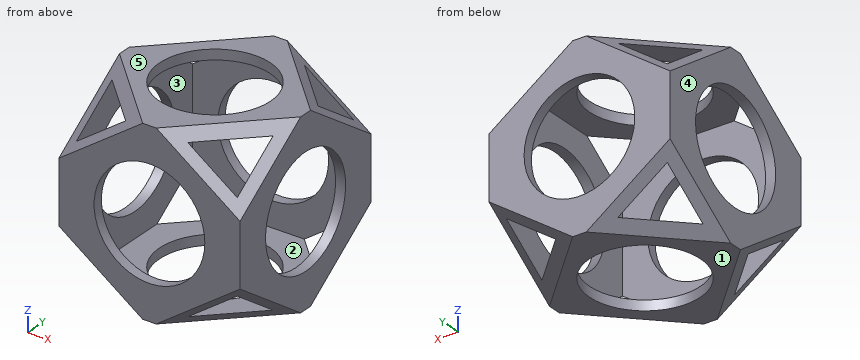
from build123d import *

# Parameters (mm, degrees)
PAD001_DEPTH            = 35
PAD_DEPTH               = 35
CYLINDER002_R           = 27.5
CYLINDER002_DEPTH       = 90
CYLINDER002_PITCH_ANGLE = 90
CYLINDER001_R           = 27.5
CYLINDER001_DEPTH       = 90
CYLINDER001_ROLL_ANGLE  = 90
CYLINDER_R              = 27.5
CYLINDER_DEPTH          = 90
BOX001_W                = 80
BOX001_H                = 80
BOX001_DEPTH            = 80
BOX_W                   = 90
BOX_H                   = 90
BOX_DEPTH               = 90


with BuildPart() as pad001:
    # Sketch001 → Pad001 (new body, symmetric)
    with BuildSketch(Plane(origin=(0, 0, 0), x_dir=(0.707107, -0.707107, 0), z_dir=(-0.707107, -0.707107, 0))):
        Polygon((-65, 14.195959), (-65, 50), (-29.195959, 50), align=None)
        Polygon((29.195959, 50), (65, 50), (65, 14.195959), align=None)
        Polygon((-65, -14.195959), (-65, -50), (-29.195959, -50), align=None)
        Polygon((29.195959, -50), (65, -50), (65, -14.195959), align=None)
    extrude(amount=PAD001_DEPTH, both=True)


with BuildPart() as pad:
    # Sketch → Pad (new body, symmetric)
    with BuildSketch(Plane(origin=(0, 0, 0), x_dir=(0.707107, 0.707107, 0), z_dir=(0.707107, -0.707107, 0))):
        Polygon((-65, 14.195959), (-65, 50), (-29.195959, 50), align=None)
        Polygon((29.195959, 50), (65, 50), (65, 14.195959), align=None)
        Polygon((-65, -14.195959), (-65, -50), (-29.195959, -50), align=None)
        Polygon((29.195959, -50), (65, -50), (65, -14.195959), align=None)
    extrude(amount=PAD_DEPTH, both=True)


with BuildPart() as cylinder002:
    # Cylinder002 → Cylinder002 (new body)
    with BuildSketch(Plane.XY):
        Circle(CYLINDER002_R)
    extrude(amount=CYLINDER002_DEPTH)


with BuildPart() as cylinder002_1:
    # Cylinder002 pitch: moved
    add(cylinder002.part.rotate(Axis((0, 0, 0), (0, 1, 0)), CYLINDER002_PITCH_ANGLE))


with BuildPart() as cylinder002_2:
    # Cylinder002 placement: moved
    add(cylinder002_1.part.moved(Location((-45, 0, 0))))


with BuildPart() as cylinder001:
    # Cylinder001 → Cylinder001 (new body)
    with BuildSketch(Plane.XY):
        Circle(CYLINDER001_R)
    extrude(amount=CYLINDER001_DEPTH)


with BuildPart() as cylinder001_1:
    # Cylinder001 roll: moved
    add(cylinder001.part.rotate(Axis((0, 0, 0), (1, 0, 0)), CYLINDER001_ROLL_ANGLE))


with BuildPart() as cylinder001_2:
    # Cylinder001 placement: moved
    add(cylinder001_1.part.moved(Location((0, 45, 0))))


with BuildPart() as cylinder:
    # Cylinder → Cylinder (new body)
    with BuildSketch(Plane.XY.offset(-45)):
        Circle(CYLINDER_R)
    extrude(amount=CYLINDER_DEPTH)


with BuildPart() as obj1:
    # Box001 → Box001 (new body)
    with BuildSketch(Plane(origin=(-40, -40, -40), x_dir=(1, 0, 0), z_dir=(0, 0, 1))):
        with Locations((40, 40)):
            Rectangle(BOX001_W, BOX001_H)
    extrude(amount=BOX001_DEPTH)


with BuildPart() as cut005:
    # Box → Box (new body)
    with BuildSketch(Plane(origin=(-45, -45, -45), x_dir=(1, 0, 0), z_dir=(0, 0, 1))):
        with Locations((45, 45)):
            Rectangle(BOX_W, BOX_H)
    extrude(amount=BOX_DEPTH)

    # Cut: cut obj1
    add(obj1.part, mode=Mode.SUBTRACT)

    # Cut001: cut Cylinder
    add(cylinder.part, mode=Mode.SUBTRACT)

    # Cut002: cut Cylinder001
    add(cylinder001_2.part, mode=Mode.SUBTRACT)

    # Cut003: cut Cylinder002
    add(cylinder002_2.part, mode=Mode.SUBTRACT)

    # Cut004: cut Pad
    add(pad.part, mode=Mode.SUBTRACT)

    # Cut005: cut Pad001
    add(pad001.part, mode=Mode.SUBTRACT)


solid = cut005.part
Geometry: final body of the model. Coordinates: model frame, mm. Face numbers are marked on the shaded views. A direction names the side the tool comes from. Coordinates: 2 decimals unless noted, no trailing zeros. Order: outer loops, then holes, each group sorted by start corner. A loop starts at its lowest first (then second) coordinate and runs counter-clockwise, first axis right, second up. Notation, with made-up numbers: M 6.25,-25 L 30.25,-25 A20 ccw 30.25,-21 Z; hole C -13.75,13.25 d3. An arc over 180 degrees is marked long. One line per question, with ' | ' between items. Start each with the question number.
Item 1: Set-up query: the marked faces 1 and 2. Return all of +Z, -Z, +X, -X, +Y, -Y with unobstructed straight access to the full face (end or side cutting, diameter ignored); none if empty.
Item 2: Draft query along X for the marked faces 3, 4 and 5. Return one class per face: released by +X, released by -X, zero draft, split by the parting line, or undercut.
Item 3: Cut plane C-C, the plane y = 38. Return the cut outline in (x, z).
Item 4: Cut plane A-A, the plane x = 0. Return the cut outline in (y, z), then the cut area to 3 significant figures.
Item 5: Cut plane D-D, the plane z = -26. Count the separate pieces of the cut face and the enclosed holes in it, then the cut area to 3 significant figures.
Item 6: Ray query, probe 1 along X at (y, z) = (42, 0); probe 2 along Z at (x, y) = (20.5, 26.5). Return the intervals inside material, ascending. Write a range as [from, to].
Item 7: Pin query (flat end, axial travel): pin 1 Ø4 at (y, z) = (-22.5, 8.5) entering from +X; pin 2 Ø1 at (x, z) = (32, 26) entering from +Y. Return the tip coordinate at first contact, or that it passes through.
A:
1) face 1: -Z, +X, -X, +Y, -Y | face 2: none
2) face 3: undercut | face 4: released by -X | face 5: zero draft
3) outline: M -45,-20.51 L -40,-24.04 L -40,24.04 L -45,20.51 Z; M -17.43,-40 L -10.36,-45 L 10.36,-45 L 17.43,-40 Z; M -17.43,40 L 17.43,40 L 10.36,45 L -10.36,45 Z; M 40,-24.04 L 45,-20.51 L 45,20.51 L 40,24.04 Z
4) outline: M -45,-45 L -27.5,-45 L -27.5,-40 L -40,-40 L -40,-27.5 L -45,-27.5 Z; M -45,27.5 L -40,27.5 L -40,40 L -27.5,40 L -27.5,45 L -45,45 Z; M 27.5,-45 L 45,-45 L 45,-27.5 L 40,-27.5 L 40,-40 L 27.5,-40 Z; M 27.5,40 L 40,40 L 40,27.5 L 45,27.5 L 45,45 L 27.5,45 Z | area: 600 mm2
5) separate pieces: 8 | enclosed holes: 0 | area: 951 mm2
6) probe 1: x = [-45, -27.5], [27.5, 45] | probe 2: z = [-45, -40], [40, 45]
7) pin 1: passes through | pin 2: stops at y = 44.1
